Autodesk Inventor part; units mm, degrees
ref_plane "YZ Plane" through (0, 0, 0) normal (1, 0, 0) x (0, 1, 0)
ref_plane "XZ Plane" through (0, 0, 0) normal (0, 1, 0) x (-1, 0, 0)
ref_plane "XY Plane" through (0, 0, 0) normal (0, 0, 1) x (1, 0, 0)
sketch "Sketch1" plane through (0, 0, 0) normal (1, 0, 0) x (0, 1, 0)
  line L0 (0, 0) -> (65.278, 0)
  line L1 (65.278, 0) -> (65.278, -16.1544)
  line L2 (0, -16.1544) -> (0, 0)
  line L3 (0, 0) -> (0, -20.066)
  line L4 (65.278, 0) -> (0, 0)
  line L5 (0, 0) -> (0, -36.5125)
  line L6 (0, -36.5125) -> (65.278, -36.5125)
  line L7 (65.278, -36.5125) -> (65.278, 0)
  dimension "d0" = 65.278
  dimension "d1" = 16.1544
  dimension "d11" = 36.5125
extrude "Extrusion1" add sketch "Sketch1" along normal blind 4.7625
sketch "Sketch3" plane through (0, 0, 0) normal (0, 0, 1) x (1, 0, 0)
  line L0 (0, 65.278) -> (0, 0)
  line L1 (0, 0) -> (4.7625, 0)
  line L2 (4.7625, 65.278) -> (4.7625, 0)
  line L3 (0, 65.278) -> (4.7625, 65.278)
  line L4 (4.7625, 65.278) -> (4.7625, 0)
  line L5 (4.7625, 65.278) -> (-21.59, 65.278)
  line L6 (-21.59, 65.278) -> (-21.59, 0)
  line L7 (-21.59, 0) -> (4.7625, 0)
  line L8 (4.7625, 0) -> (4.7625, 65.278)
  dimension "d12" = 26.3525
extrude "Extrusion3" add sketch "Sketch3" against normal blind 4.7625 contours L0 L7 L6 L5
sketch "Sketch4" plane through (0, 65.278, -36.5125) normal (0, 1, 0) x (1, 0, 0)
  line L0 (0, 0) -> (0, -31.75)
  line L1 (-21.59, -31.75) -> (0, -31.75)
  line L2 (-21.59, -36.5125) -> (-21.59, -31.75)
  line L3 (4.7625, -36.5125) -> (-21.59, -36.5125)
  line L4 (4.7625, 0) -> (4.7625, -36.5125)
  line L5 (0, 0) -> (4.7625, 0)
  line L6 (-21.59, -31.75) -> (0, -31.75)
  line L7 (-21.59, -31.75) -> (-21.59, 0)
  line L8 (0, 0) -> (-21.59, 0)
  line L9 (-21.59, 0) -> (0, 0)
  line L10 (0, 0) -> (0, -31.75)
  line L11 (0, -31.75) -> (-21.59, -31.75)
  line L12 (-21.59, -31.75) -> (-21.59, 0)
  point P0 (0, -36.5125)
  dimension "d15" = 31.75
  dimension "d16" = 21.59
  dimension "d50" = 31.75
  dimension "d51" = 21.59
extrude "Extrusion4" add sketch "Sketch4" against normal blind 4.7625
fillet "Fillet1" radius 1.5875 3 edges at (0, 60.5155, -20.6375) (-10.795, 60.5155, -4.7625) (0, 30.2578, -4.7625)
sketch "Sketch6" plane through (0, 0, -36.5125) normal (0, -1, 0) x (1, 0, 0)
  line L0 (0, 30.1625) -> (0, 0)
  line L1 (0, 0) -> (4.7625, 0)
  line L2 (4.7625, 36.5125) -> (4.7625, 0)
  line L3 (-21.59, 36.5125) -> (4.7625, 36.5125)
  line L4 (-21.59, 36.5125) -> (-21.59, 31.75)
  line L5 (-1.5875, 31.75) -> (-21.59, 31.75)
  arc A0 (0, 30.1625) -> (-1.5875, 31.75) centre (-1.5875, 30.1625) ccw
  line L6 (0, 0) -> (9.525, 0)
  line L7 (9.525, 0) -> (9.525, 9.525)
  line L8 (9.525, 9.525) -> (0, 9.525)
  line L9 (0, 9.525) -> (0, 0)
  line L10 (-21.59, 36.5125) -> (-21.59, 31.75)
  line L11 (-21.59, 31.75) -> (-12.065, 31.75)
  line L12 (-12.065, 31.75) -> (-12.065, 41.275)
  line L13 (-12.065, 41.275) -> (-21.59, 41.275)
  line L14 (-21.59, 41.275) -> (-21.59, 31.75)
  point P0 (0, 36.5125)
  dimension "d24" = 9.525
  dimension "d25" = 9.525
  dimension "d26" = 9.525
  dimension "d27" = 9.525
extrude "Extrusion5" add sketch "Sketch6" against normal blind 12.7 contours L8 L2 L1 L0 | L8 L7 L6 L2 | L5 L4 L3 L12 | L3 L14 L13 L12
chamfer "Chamfer1" distance 4.7625 angle 45 4 edges at (4.7625, 6.35, -26.9875) (-12.065, 6.35, 0) (4.7625, 12.7, -31.75) (-16.8275, 12.7, 0)
sketch "Sketch8" plane through (-21.59, 0, -4.7625) normal (0, -1, 0) x (1, 0, 0)
  line L0 (20.0025, 0) -> (0, 0)
  arc A0 (21.59, -1.5875) -> (20.0025, 0) centre (20.0025, -1.5875) ccw
  line L1 (21.59, -1.5875) -> (21.59, -31.75)
  line L2 (21.59, -31.75) -> (31.115, -31.75)
  line L3 (31.115, -31.75) -> (31.115, -22.225)
  line L4 (26.3525, -17.4625) -> (31.115, -22.225)
  line L5 (26.3525, 4.7625) -> (26.3525, -17.4625)
  line L6 (14.2875, 4.7625) -> (26.3525, 4.7625)
  line L7 (9.525, 9.525) -> (14.2875, 4.7625)
  line L8 (9.525, 9.525) -> (0, 9.525)
  line L9 (0, 9.525) -> (0, 0)
  line L10 (26.3525, 4.7625) -> (0, 4.7625)
  point P0 (21.59, 4.7625)
  point P1 (4.7625, 4.7625)
  point P2 (26.3525, -26.9875)
hole "Hole1" at (-16.8275, 0, 0) at (4.7625, 0, -31.75) direction (0, 1, 0) diameter 2.6416 depth 12.7 tip angle 118
sketch "Sketch9" plane through (4.7625, 65.278, 0) normal (0, 1, 0) x (1, 0, 0)
  line L0 (-26.3525, 36.5125) -> (0, 36.5125)
  line L1 (-26.3525, 0) -> (-26.3525, 36.5125)
  line L2 (0, 0) -> (-26.3525, 0)
  line L3 (0, 36.5125) -> (0, 0)
  point P0 (-4.7625, 0)
  point P1 (-20.0025, 6.35)
  point P2 (-16.1925, 26.3525)
  dimension "d52" = 6.35
  dimension "d56" = 10.16
  dimension "d57" = 6.35
  dimension "d58" = 10.16
hole "Hole2" at (-15.24, 65.278, -6.35) at (-11.43, 65.278, -26.3525) direction (0, -1, 0) diameter 2.6416 end through all
fillet "Fillet2" radius 6.35 1 edges at (-21.59, 62.8968, -36.5125)
equation "\"d15\" = d50"
equation "\"d16\" = d51"
properties part number "WheelIntakeBrace"
Check sheet for the modelled part. Datum: model origin and axes. Units: mm. A direction names the side the tool comes from. Give positions to 0.01 mm unless a question says otherwise; leave off trailing zeros. Order: outer loops, then holes, each group sorted by start corner. A loop starts at its lowest first (then second) coordinate and runs counter-clockwise, first axis right, second up. Notation, with made-up numbers: (-39.75, -20) -> (-27.75, -20) arc R20 cw to (-27.75, 12) -> close; hole circle Ø3 at (83, 37.5). An arc over 180 degrees is marked (long way). Use CSV: the item, a comma, the result in double quotes. Start each with the question number.
1) Set-up check for faces 4 (the face through (-0.45, 29.05, -5.24)), 5 (the face through (4.762, 32, -18)), 6 (the face through (-17.72, 6.439, 0.973)): record each of +Z, -Z, +X, -X, +Y, -Y from which the full face is reachable in a straight line by a thin tool's end or side.
2) Sectioned sample at C-C, the plane y = 8. Give the number of separate pieces and of enclosed holes in the cut face, plus the area to 3 significant figures.
3) Mould release check, pull along Z, two halves, no side actions. Record for faces 1 (the face through (7.177, 6.669, -24.64)), 2 (the face through (-15.64, 62.51, -5.09)), 3 (the face through (-12, 30, -4.762)): released by +Z, released by -Z, zero draft, split by the parting line, or undercut.
4) Sectioned sample at B-B, the plane z = -10.5. Record the boundary of the cut face in (x, y) (1 decimal).
5) Go/stop test with flat-tipped pins: P1, Ø5, axis at y = 29.5, z = -12.5, coming from the +X side; P2, Ø1.5, axis at x = -6.5, y = 41, coming from the -Z side; P3, Ø24, axis at y = 29.5, z = -22, coming from the -X side. Record where each tip stops, or that it passes through.
6) Material ranges on line 1 (X direction, y = 3.5, z = -31.75) (3 decimals); line 2 (Z direction, x = -15.24, y = 63.8); line 3 (Y direction, x = -1.5, z = -24.5), recorded low to high. Write a range as from..to.
Recorded:
1,face 4,"-Z, -X, -Y"
1,face 5,"+Z, +X, +Y"
1,face 6,"-Y"
2,separate pieces,"1"
2,enclosed holes,"2"
2,area,"380 mm2"
3,face 1,"released by +Z"
3,face 2,"undercut"
3,face 3,"released by -Z"
4,outline,"(-21.6, 60.5) -> (-1.6, 60.5) arc R1.6 cw to (0, 58.9) -> (0, 0) -> (4.8, 0) -> (4.8, 65.3) -> (-21.6, 65.3) -> close"
5,P1,"x = 4.76"
5,P2,"z = -4.76"
5,P3,"x = 0"
6,line 1,"0..3.442, 6.083..9.525"
6,line 2,"-36.51..-7.67, -5.03..0"
6,line 3,"60.51..65.28"
